```python
from build123d import *

# Parameters (mm, degrees)
SKETCH1_W                         = 152.4
SKETCH1_H                         = 101.6
BOSS_EXTRUDE1_DEPTH               = 12.7
SKETCH2_W                         = 101.6
SKETCH2_H                         = 101.6
BOSS_EXTRUDE2_DEPTH               = 76.2
SKETCH3_W                         = 76.2
SKETCH3_H                         = 76.2
CUT_EXTRUDE1_DEPTH                = 76.2
SKETCH4_R                         = 31.75
BOSS_EXTRUDE3_DEPTH               = 6.35
SKETCH5_R                         = 25.4
CUT_EXTRUDE2_DEPTH                = 164.628053829
CIRPATTERN1_COUNT                 = 6
FILLET1_R                         = 6.35
F_1_4_20_TAPPED_HOLE1_D           = 5.1054
F_1_4_20_TAPPED_HOLE1_DEPTH       = 19.05
F_1_4_20_TAPPED_HOLE1_CSINK_D     = 7.62
F_1_4_20_TAPPED_HOLE1_CSINK_ANGLE = 90
F_1_4_20_TAPPED_HOLE1_TIP         = 1.533816902
CUT_EXTRUDE3_DEPTH                = 122.979516723
LPATTERN1_COUNT                   = 2
LPATTERN1_PITCH                   = 63.5
MIRROR3_COPY_1_DEPTH              = 122.979516723


with BuildPart() as part:
    # Sketch1 → Boss-Extrude1 (new body)
    with BuildSketch(Plane(origin=(0, 0, 0), x_dir=(1, 0, 0), z_dir=(0, 1, 0))):
        Rectangle(SKETCH1_W, SKETCH1_H)
    extrude(amount=BOSS_EXTRUDE1_DEPTH)

    # Sketch2 → Boss-Extrude2 (add)
    with BuildSketch(Plane(origin=(0, 12.7, 0), x_dir=(1, 0, 0), z_dir=(0, 1, 0))):
        Rectangle(SKETCH2_W, SKETCH2_H)
    extrude(amount=BOSS_EXTRUDE2_DEPTH)

    # Sketch3 → Cut-Extrude1 (cut)
    with BuildSketch(Plane(origin=(0, 88.9, 0), x_dir=(1, 0, 0), z_dir=(0, 1, 0))):
        Rectangle(SKETCH3_W, SKETCH3_H)
    extrude(amount=-CUT_EXTRUDE1_DEPTH, mode=Mode.SUBTRACT)

    # Sketch4 → Boss-Extrude3 (add)
    with BuildSketch(Plane.XY.offset(50.8)):
        with Locations((0, 44.45)):
            Circle(SKETCH4_R)
    boss_extrude3 = extrude(amount=BOSS_EXTRUDE3_DEPTH)

    # Mirror1: Boss-Extrude3 across plane
    add(boss_extrude3.mirror(Plane.XY))

    # Sketch5 → Cut-Extrude2 (cut, through all)
    with BuildSketch(Plane.XY.offset(57.15)):
        with Locations((0, 44.45)):
            Circle(SKETCH5_R)
    extrude(amount=-CUT_EXTRUDE2_DEPTH, mode=Mode.SUBTRACT)

    # Sketch7 → #4-40 Tapped Hole1 (revolve, cut)
    with BuildSketch(Plane(origin=(14.2875, 69.196675913, 57.15), x_dir=(0, -1, 0), z_dir=(1, 0, 0))):
        Polygon((0, 0), (0, 9.569152758), (1.1303, 8.89), (1.1303, 0.9271), (2.0574, 0), align=None)
    f_4_40_tapped_hole1 = revolve(axis=Axis((14.2875, 69.196675913, 63.5), (0, 0, -1)), mode=Mode.SUBTRACT)

    # CirPattern1: #4-40 Tapped Hole1 ×6 about axis
    cirpattern1_axis = Axis((0, 44.45, 0), (0, 0, 1))
    for i in range(1, CIRPATTERN1_COUNT):
        add(f_4_40_tapped_hole1.rotate(cirpattern1_axis, i * 360 / CIRPATTERN1_COUNT), mode=Mode.SUBTRACT)

    # Mirror2: #4-40 Tapped Hole1 across plane
    add(f_4_40_tapped_hole1.mirror(Plane.XY), mode=Mode.SUBTRACT)

    # Mirror2 copy 1 sketch → Mirror2 copy 1 (revolve, cut)
    with BuildSketch(Plane(origin=(-14.2875, 69.196675913, -57.15), x_dir=(0.8660254037844386, -0.5000000000000001, 0), z_dir=(0.5000000000000001, 0.8660254037844386, 0))):
        Polygon((0, 0), (0, -9.569152758), (1.1303, -8.89), (1.1303, -0.9271), (2.0574, 0), align=None)
    revolve(axis=Axis((-14.2875, 69.196675913, -63.5), (0, 0, -1)), mode=Mode.SUBTRACT)

    # Mirror2 copy 2 sketch → Mirror2 copy 2 (revolve, cut)
    with BuildSketch(Plane(origin=(-28.575, 44.45, -57.15), x_dir=(0.8660254037844387, 0.4999999999999998, 0), z_dir=(-0.4999999999999998, 0.8660254037844387, 0))):
        Polygon((0, 0), (0, -9.569152758), (1.1303, -8.89), (1.1303, -0.9271), (2.0574, 0), align=None)
    revolve(axis=Axis((-28.575, 44.45, -63.5), (0, 0, -1)), mode=Mode.SUBTRACT)

    # Mirror2 copy 3 sketch → Mirror2 copy 3 (revolve, cut)
    with BuildSketch(Plane(origin=(-14.2875, 19.703324087, -57.15), x_dir=(0, 1, 0), z_dir=(-1, 0, 0))):
        Polygon((0, 0), (0, -9.569152758), (1.1303, -8.89), (1.1303, -0.9271), (2.0574, 0), align=None)
    revolve(axis=Axis((-14.2875, 19.703324087, -63.5), (0, 0, -1)), mode=Mode.SUBTRACT)

    # Mirror2 copy 4 sketch → Mirror2 copy 4 (revolve, cut)
    with BuildSketch(Plane(origin=(14.2875, 19.703324087, -57.15), x_dir=(-0.8660254037844384, 0.5000000000000004, 0), z_dir=(-0.5000000000000004, -0.8660254037844384, 0))):
        Polygon((0, 0), (0, -9.569152758), (1.1303, -8.89), (1.1303, -0.9271), (2.0574, 0), align=None)
    revolve(axis=Axis((14.2875, 19.703324087, -63.5), (0, 0, -1)), mode=Mode.SUBTRACT)

    # Mirror2 copy 5 sketch → Mirror2 copy 5 (revolve, cut)
    with BuildSketch(Plane(origin=(28.575, 44.45, -57.15), x_dir=(-0.8660254037844386, -0.5000000000000001, 0), z_dir=(0.5000000000000001, -0.8660254037844386, 0))):
        Polygon((0, 0), (0, -9.569152758), (1.1303, -8.89), (1.1303, -0.9271), (2.0574, 0), align=None)
    revolve(axis=Axis((28.575, 44.45, -63.5), (0, 0, -1)), mode=Mode.SUBTRACT)

    # Fillet1
    fillet1_edges = [part.edges().sort_by_distance(p)[0] for p in [
        (50.8, 50.8, 50.8),
        (50.8, 50.8, -50.8),
        (-50.8, 50.8, -50.8),
        (-50.8, 50.8, 50.8),
    ]]
    fillet(fillet1_edges, radius=FILLET1_R)

    # 1/4-20 Tapped Hole1
    with Locations(Plane(origin=(0, 88.9, 0), x_dir=(1, 0, 0), z_dir=(0, 1, 0))):
        with Locations((-44.45, 44.45), (44.45, 44.45), (44.45, -44.45), (-44.45, -44.45)):
            CounterSinkHole(F_1_4_20_TAPPED_HOLE1_D / 2, F_1_4_20_TAPPED_HOLE1_CSINK_D / 2, depth=F_1_4_20_TAPPED_HOLE1_DEPTH, counter_sink_angle=F_1_4_20_TAPPED_HOLE1_CSINK_ANGLE)
            with Locations((0, 0, -(F_1_4_20_TAPPED_HOLE1_DEPTH + F_1_4_20_TAPPED_HOLE1_TIP / 2))):  # 118° drill point
                Cone(0, F_1_4_20_TAPPED_HOLE1_D / 2, F_1_4_20_TAPPED_HOLE1_TIP, mode=Mode.SUBTRACT)

    # Sketch12 → Cut-Extrude3 (cut, through all)
    with BuildSketch(Plane(origin=(0, 12.7, 0), x_dir=(1, 0, 0), z_dir=(0, 1, 0))):
        with BuildLine():
            Line((66.675, -25.4), (66.675, -38.1))
            ThreePointArc((66.675, -38.1), (63.5, -41.275), (60.325, -38.1))
            Line((60.325, -38.1), (60.325, -25.4))
            ThreePointArc((60.325, -25.4), (63.5, -22.225), (66.675, -25.4))
        make_face()
    cut_extrude3 = extrude(amount=-CUT_EXTRUDE3_DEPTH, mode=Mode.SUBTRACT)

    # LPattern1: Cut-Extrude3 ×2
    with Locations(*[(0, 0, -i * LPATTERN1_PITCH) for i in range(1, LPATTERN1_COUNT)]):
        add(cut_extrude3, mode=Mode.SUBTRACT)

    # Mirror3: Cut-Extrude3 across plane
    add(cut_extrude3.mirror(Plane(origin=(0, 0, 0), x_dir=(0, 0, 1), z_dir=(1, 0, 0))), mode=Mode.SUBTRACT)

    # Mirror3 copy 1 sketch → Mirror3 copy 1 (cut, through all)
    with BuildSketch(Plane(origin=(0, 12.7, -63.5), x_dir=(-1, 0, 0), z_dir=(0, 1, 0))):
        with BuildLine():
            Line((66.675, 25.4), (66.675, 38.1))
            ThreePointArc((66.675, 38.1), (63.5, 41.275), (60.325, 38.1))
            Line((60.325, 38.1), (60.325, 25.4))
            ThreePointArc((60.325, 25.4), (63.5, 22.225), (66.675, 25.4))
        make_face()
    extrude(amount=-MIRROR3_COPY_1_DEPTH, mode=Mode.SUBTRACT)


solid = part.part
```
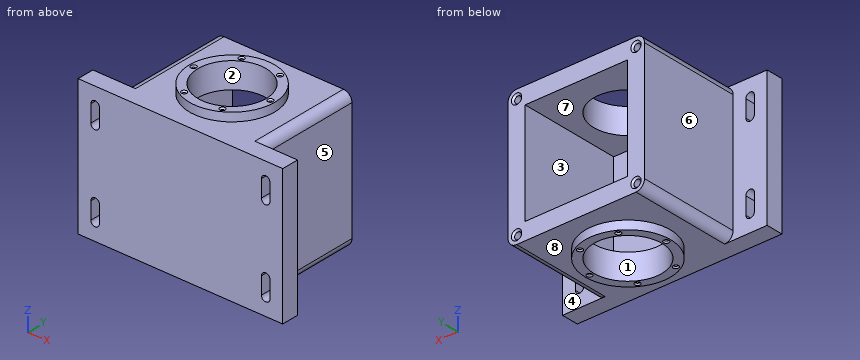
Build history of the part. All positions in model axes, mm. Face numbers are marked on the shaded views. A direction names the side the tool comes from. Round coordinates to 2 decimals unless told otherwise and drop trailing zeros. Write each loop counter-clockwise with the first axis right and the second up, starting at its lowest first coordinate (ties: lowest second). Pieces come first, ordered by that corner, then holes. Notation, with made-up numbers: (78.5, -18.5) - (84.5, -18.5) arc R26 cw to (84.5, -0.5) - close; hole circle Ø11 at (-6, -23.5). An arc over 180 degrees is marked (long way). Answer as CSV lines item,"result".
Q1. Drill centre lines: probe 1 along X at (y, z) = (77, -44); probe 2 along X at (y, z) = (68.5, -22); probe 3 along X at (y, z) = (44, 52). Where is each one in solid material? Low to high. Write a range as [from, to].
Report:
probe 1,"x = [-50.8, -46.96], [-41.94, 41.94], [46.96, 50.8]"
probe 2,"x = [-50.8, -38.1], [38.1, 50.8]"
probe 3,"x = [-31.75, -29.61], [-27.54, -25.4], [25.4, 27.54], [29.61, 31.75]"
Q2. Pull direction Y, two halves, no side cores. Call the marked faces 1, 2, 3 and 4: +Y half, -Y half, draft (parallel to the pull), parting line (faces both ways), or undercut.
Report:
face 1,"undercut"
face 2,"undercut"
face 3,"draft"
face 4,"+Y half"
Q3. Tool access for the marked faces 5, 6, 7 and 8: list every direction of +Z, -Z, +X, -X, +Y, -Y with a clear straight run to the whole face (end or side of a thin tool).
Report:
face 5,"+Z, -Z, +X, +Y"
face 6,"+Z, -Z, -X, +Y"
face 7,"+Y"
face 8,"-Z"
Q4. Cut at B-B (y = 29). Write the cut outline in (x, z).
Report:
outline,"(-50.8, -44.45) arc R6.35 ccw to (-44.45, -50.8) - (-27.74, -50.8) - (-27.74, -57.15) - (-20.16, -57.15) - (-20.16, -38.1) - (-38.1, -38.1) - (-38.1, 38.1) - (-20.16, 38.1) - (-20.16, 57.15) - (-27.74, 57.15) - (-27.74, 50.8) - (-44.45, 50.8) arc R6.35 ccw to (-50.8, 44.45) - close; (20.16, -57.15) - (27.74, -57.15) - (27.74, -50.8) - (44.45, -50.8) arc R6.35 ccw to (50.8, -44.45) - (50.8, 44.45) arc R6.35 ccw to (44.45, 50.8) - (27.74, 50.8) - (27.74, 57.15) - (20.16, 57.15) - (20.16, 38.1) - (38.1, 38.1) - (38.1, -38.1) - (20.16, -38.1) - close"
Q5. Cut at A-A (x = 63.5). Write the cut outline in (y, z) (3 decimals), and give its area (3 significant figures).
Report:
outline,"(0, -50.8) - (12.7, -50.8) - (12.7, -41.275) - (0, -41.275) - close; (0, -22.225) - (12.7, -22.225) - (12.7, 22.225) - (0, 22.225) - close; (0, 41.275) - (12.7, 41.275) - (12.7, 50.8) - (0, 50.8) - close"
area,"806 mm^2"
Q6. Cut at C-C (z = 3). Write the cut outline in (x, y), and give its area (3 significant figures).
Report:
outline,"(-76.2, 0) - (76.2, 0) - (76.2, 12.7) - (50.8, 12.7) - (50.8, 88.9) - (38.1, 88.9) - (38.1, 12.7) - (-38.1, 12.7) - (-38.1, 88.9) - (-50.8, 88.9) - (-50.8, 12.7) - (-76.2, 12.7) - close"
area,"3,870 mm^2"
Q7. Cut at D-D (x = 0). Write the cut outline in (y, z).
Report:
outline,"(0, -50.8) - (12.7, -50.8) - (12.7, -57.15) - (19.05, -57.15) - (19.05, -38.1) - (12.7, -38.1) - (12.7, 38.1) - (19.05, 38.1) - (19.05, 57.15) - (12.7, 57.15) - (12.7, 50.8) - (0, 50.8) - close; (69.85, -57.15) - (76.2, -57.15) - (76.2, -50.8) - (88.9, -50.8) - (88.9, -38.1) - (69.85, -38.1) - close; (69.85, 38.1) - (88.9, 38.1) - (88.9, 50.8) - (76.2, 50.8) - (76.2, 57.15) - (69.85, 57.15) - close"
Q8. Drop flat-ended pins along their axis: pin 1 (2 mm diameter, centred on x = 14.29, y = 19.7, fed in from -Z); pin 2 (3 mm diameter, centred on x = -14.29, y = 69.2, fed in from +Z); pin 3 (10 mm diameter, centred on x = -59.5, y = 17, fed in from +Z). Give the stop position or say it passes through.
Report:
pin 1,"stops at z = -48.18"
pin 2,"stops at z = 56.6"
pin 3,"stops at z = 50.8"
